Design review of the part built by this model. Coordinates are the model's own, in mm. Face numbers are marked on the shaded views. A direction names the side the tool comes from. Coordinates: 2 decimals unless noted, no trailing zeros. Write each loop counter-clockwise with the first axis right and the second up, starting at its lowest first coordinate (ties: lowest second). Pieces come first, ordered by that corner, then holes. Notation, with made-up numbers: (72.25, 78) -> (104.25, 78) arc R14 ccw to (104.25, 101) -> close; hole circle Ø8 at (70.25, 41). An arc over 180 degrees is marked (long way). Answer in a Markdown table with one row per item. Add a question column.
Item 1: Take a section at C-C, the plane x = -18. Give the number of separate pieces and of enclosed holes in the cut face, and give its area (3 significant figures).
Item 2: Take a section at A-A, the plane z = 0. Write out the cut boundary in (x, y) (3 decimals), and give its area (3 significant figures).
Item 3: Take a section at B-B, the plane y = 41. Write out the cut boundary in (x, z), and give its area (3 significant figures).
Item 4: For the marked faces 5 and 6, list the 3-axis set-ups (+Z, -Z, +X, -X, +Y, -Y) from which the entire face can be reached by the end or side of a thin tool; tool diameter is ignored.
Item 5: Draft analysis for pull direction X (two halves, no side actions). For the marked faces 1, 2, 3 and 4, state which applies: released by +X, released by -X, zero draft, split by the parting line, or undercut.
Item 6: Clearance check with flat-ended pins moving along their axes: P1, Ø6, axis at y = 38, z = 44.5, coming from the -X side; P2, Ø2, axis at y = 12.5, z = 44.5, coming from the +X side; P3, Ø12, axis at x = 41, y = 9, coming from the +Z side. State where each tip first meets the part, or that it passes through.
Item 7: To check wall thickness, follow line 1 (X direction, y = 0.8, z = -42); line 2 (Y direction, x = 49, z = -22); line 3 (Z direction, x = -14.5, y = 52.5). State the ranges of each line that lie inside material, in increasing order.
from build123d import *

# Parameters (mm, degrees)
SKETCH1_R                                           = 60.625
SKETCH1_R_2                                         = 45
BOSS_EXTRUDE1_DEPTH                                 = 4
SKETCH2_R                                           = 49
SKETCH2_R_2                                         = 45
BOSS_EXTRUDE2_DEPTH                                 = 52
SKETCH3_W                                           = 8
SKETCH3_H                                           = 38
BOSS_EXTRUDE3_DEPTH                                 = 13
SKETCH6_W                                           = 10
SKETCH6_H                                           = 24
CUT_EXTRUDE1_DEPTH                                  = 26
SKETCH7_R                                           = 5
CUT_EXTRUDE2_DEPTH                                  = 58
SKETCH8_R                                           = 1.3
CUT_EXTRUDE3_DEPTH                                  = 7.2
BOSS_EXTRUDE4_DEPTH                                 = 4
CSK_FOR_M3_COUNTERSUNK_FLAT_HEAD_SCREW1_D           = 3.4
CSK_FOR_M3_COUNTERSUNK_FLAT_HEAD_SCREW1_DEPTH       = 4
CSK_FOR_M3_COUNTERSUNK_FLAT_HEAD_SCREW1_CSINK_D     = 6.3
CSK_FOR_M3_COUNTERSUNK_FLAT_HEAD_SCREW1_CSINK_ANGLE = 90
CSK_FOR_M3_COUNTERSUNK_FLAT_HEAD_SCREW1_TIP         = 1.021463052
FILLET1_R                                           = 1


with BuildPart() as part:
    # Sketch1 → Boss-Extrude1 (new body)
    with BuildSketch(Plane(origin=(0, 0, 0), x_dir=(1, 0, 0), z_dir=(0, 1, 0))):
        with Locations(Location((0, 0, 0), (0, 0, 270))):
            Circle(SKETCH1_R)
        with Locations(Location((0, 0, 0), (0, 0, 270))):
            Circle(SKETCH1_R_2, mode=Mode.SUBTRACT)
    extrude(amount=BOSS_EXTRUDE1_DEPTH)

    # Sketch2 → Boss-Extrude2 (add)
    with BuildSketch(Plane(origin=(0, 4, 0), x_dir=(1, 0, 0), z_dir=(0, 1, 0))):
        with Locations(Location((0, 0, 0), (0, 0, 90))):
            Circle(SKETCH2_R)
        with Locations(Location((0, 0, 0), (0, 0, 270))):
            Circle(SKETCH2_R_2, mode=Mode.SUBTRACT)
    extrude(amount=BOSS_EXTRUDE2_DEPTH)

    # Sketch3 → Boss-Extrude3 (add, symmetric)
    with BuildSketch(Plane(origin=(0, 0, 0), x_dir=(0, 0, -1), z_dir=(1, 0, 0))):
        with Locations((15.25, 19)):
            Rectangle(SKETCH3_W, SKETCH3_H)
        Polygon((-45, 38), (-45, 30), (-39.75, 30), (-31.75, 38), align=None)
        Polygon((-39.75, 30), (-45, 30), (-45, 24.75), align=None)
        Polygon((-31.75, 38), (-39.75, 30), (-31.75, 30), align=None)
    extrude(amount=BOSS_EXTRUDE3_DEPTH, both=True)


with BuildPart() as boss_extrude3_piece_1:
    # of the separate pieces the step leaves, piece 1, a body of its own (boss_extrude3_pieces)
    add(part.part.solids().sort_by_distance((0, 0, 60.625))[0])

    # Sketch7 → Cut-Extrude2 (cut)
    with BuildSketch(Plane.XY.offset(-11.25)):
        with Locations(Location((0, 14, 0), (0, 0, 90))):
            Circle(SKETCH7_R)
    extrude(amount=-CUT_EXTRUDE2_DEPTH, mode=Mode.SUBTRACT)


with BuildPart() as boss_extrude3_piece_2:
    # of the separate pieces the step leaves, piece 2, a body of its own (boss_extrude3_pieces)
    add(part.part.solids().sort_by_distance((-13, 38, -19.25))[0])

    # Sketch6 → Cut-Extrude1 (cut)
    with BuildSketch(Plane.XY.offset(-11.25)):
        with Locations((0, 17)):
            Rectangle(SKETCH6_W, SKETCH6_H)
    extrude(amount=-CUT_EXTRUDE1_DEPTH, mode=Mode.SUBTRACT)


with BuildPart() as cut_extrude3_tool:
    # Sketch8 → Cut-Extrude3 (new body)
    with BuildSketch(Plane(origin=(0, 38, 0), x_dir=(1, 0, 0), z_dir=(0, 1, 0))):
        with Locations(Location((-5, 13.75, 0), (0, 0, 270))):
            Circle(SKETCH8_R)
        with Locations(Location((5, 13.75, 0), (0, 0, 270))):
            Circle(SKETCH8_R)
        with Locations(Location((-5, -34.25, 0), (0, 0, 270))):
            Circle(SKETCH8_R)
        with Locations(Location((5, -34.25, 0), (0, 0, 270))):
            Circle(SKETCH8_R)
    extrude(amount=-CUT_EXTRUDE3_DEPTH)


with BuildPart() as boss_extrude3_piece_1_1:
    add(boss_extrude3_piece_1.part)

    # Cut-Extrude3: cut by cut_extrude3_tool
    add(cut_extrude3_tool.part, mode=Mode.SUBTRACT)



with BuildPart() as boss_extrude3_piece_2_1:
    add(boss_extrude3_piece_2.part)

    # Cut-Extrude3: cut by cut_extrude3_tool
    add(cut_extrude3_tool.part, mode=Mode.SUBTRACT)


with BuildPart() as boss_extrude3_piece_1_2:
    add(boss_extrude3_piece_1_1.part)

    add(boss_extrude3_piece_2_1.part)  # Boss-Extrude4 merges Boss-Extrude3 piece 2
    # Sketch9 → Boss-Extrude4 (add)
    with BuildSketch(Plane.XZ):
        with BuildLine():
            Line((13, -11.25), (-13, -11.25))
            Line((-13, -11.25), (-37.248431585, -25.249838503))
            ThreePointArc((-37.248431585, -25.249838503), (0, -45), (37.248431585, -25.249838503))
            Line((37.248431585, -25.249838503), (13, -11.25))
        make_face()
        with BuildLine():
            Line((-19.516660498, -24.25), (-24.906460381, -27.361802413))
            ThreePointArc((-24.906460381, -27.361802413), (0, -37), (24.906460381, -27.361802413))
            Line((24.906460381, -27.361802413), (19.516660498, -24.25))
            Line((19.516660498, -24.25), (-19.516660498, -24.25))
        make_face(mode=Mode.SUBTRACT)
    extrude(amount=-BOSS_EXTRUDE4_DEPTH)

    # CSK for M3 Countersunk Flat Head Screw1
    with Locations(Plane(origin=(0, 4, 0), x_dir=(1, 0, 0), z_dir=(0, 1, 0))):
        with Locations((-35, 42), (35, 42), (35, -42), (-35, -42)):
            CounterSinkHole(CSK_FOR_M3_COUNTERSUNK_FLAT_HEAD_SCREW1_D / 2, CSK_FOR_M3_COUNTERSUNK_FLAT_HEAD_SCREW1_CSINK_D / 2, depth=CSK_FOR_M3_COUNTERSUNK_FLAT_HEAD_SCREW1_DEPTH, counter_sink_angle=CSK_FOR_M3_COUNTERSUNK_FLAT_HEAD_SCREW1_CSINK_ANGLE)
            with Locations((0, 0, -(CSK_FOR_M3_COUNTERSUNK_FLAT_HEAD_SCREW1_DEPTH + CSK_FOR_M3_COUNTERSUNK_FLAT_HEAD_SCREW1_TIP / 2))):  # 118° drill point
                Cone(0, CSK_FOR_M3_COUNTERSUNK_FLAT_HEAD_SCREW1_D / 2, CSK_FOR_M3_COUNTERSUNK_FLAT_HEAD_SCREW1_TIP, mode=Mode.SUBTRACT)

    # Fillet1
    fillet1_edges = [boss_extrude3_piece_1_2.edges().sort_by_distance(p)[0] for p in [
        (0, 4, 49),
    ]]
    fillet(fillet1_edges, radius=FILLET1_R)


solid = boss_extrude3_piece_1_2.part
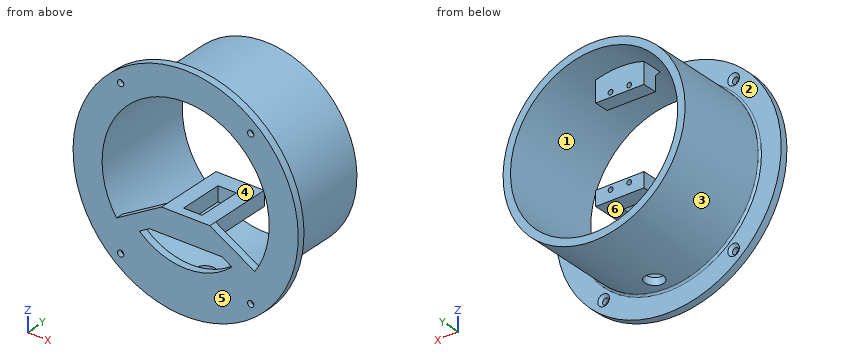
Answers:
| question | item | result |
|---|---|---|
| 1 | separate pieces | 3 |
| 1 | enclosed holes | 0 |
| 1 | area | 660 mm^2 |
| 2 | outline | (-60.625, 0) -> (-45, 0) -> (-45, 56) -> (-49, 56) -> (-49, 5) arc R1 cw to (-50, 4) -> (-60.625, 4) -> close; (45, 0) -> (60.625, 0) -> (60.625, 4) -> (50, 4) arc R1 cw to (49, 5) -> (49, 56) -> (45, 56) -> close |
| 2 | area | 541 mm^2 |
| 3 | outline | circle Ø98 at (0, 0); hole circle Ø90 at (0, 0) |
| 3 | area | 1,180 mm^2 |
| 4 | face 5 | +Z, -Z, +X, -X, -Y |
| 4 | face 6 | +Y |
| 5 | face 1 | undercut |
| 5 | face 2 | zero draft |
| 5 | face 3 | split by the parting line |
| 5 | face 4 | undercut |
| 6 | P1 | stops at x = -26.05 |
| 6 | P2 | stops at x = 22.56 |
| 6 | P3 | stops at z = 47.49 |
| 7 | line 1 | x = -43.72 to -36.7, -33.3 to 33.3, 36.7 to 43.72 |
| 7 | line 2 | y = 0 to 4 |
| 7 | line 3 | z = -46.81 to -42.6, 42.6 to 46.81 |
